from build123d import *

# Parameters (mm, degrees)
BOSS_EXTRUDE1_DEPTH      = 10
BOSS_EXTRUDE1_DEPTH_BACK = 0.01
SKETCH3_W                = 38
SKETCH3_H                = 54
CUT_EXTRUDE1_DEPTH       = 3
SKETCH5_W                = 38
SKETCH5_H                = 54
CUT_EXTRUDE3_DEPTH       = 3
SKETCH15_W               = 20
SKETCH15_H               = 50
BOSS_EXTRUDE3_DEPTH      = 20.3
SKETCH21_R               = 9
CUT_EXTRUDE21_DEPTH      = 20
SKETCH28_W               = 4.75290021
SKETCH28_H               = 9.947843747
BOSS_EXTRUDE6_DEPTH      = 115.870057685
SKETCH30_W               = 14.12
SKETCH30_H               = 25
CUT_EXTRUDE25_DEPTH      = 4.5
SKETCH33_R               = 1.55
CUT_EXTRUDE26_DEPTH      = 10.01
SKETCH36_W               = 38
SKETCH36_H               = 2
BOSS_EXTRUDE7_DEPTH      = 37
SKETCH39_R               = 6
SKETCH39_R_2             = 1.55
CUT_EXTRUDE28_DEPTH      = 2
SKETCH42_R               = 6
SKETCH42_R_2             = 1.55
CUT_EXTRUDE29_DEPTH      = 2
BOSS_EXTRUDE8_REACH      = 265.623
SKETCH44_W               = 25.175895627
SKETCH44_H               = 35.827236085


with BuildPart() as part:
    # Sketch1 → Boss-Extrude1 (new, two sides: drawn at the far end of the back side and taken through both)
    with BuildSketch(Plane.XY.offset(-BOSS_EXTRUDE1_DEPTH_BACK)):
        with BuildLine():
            Line((0, 0), (0, -37))
            Line((0, -37), (60, -37))
            Line((60, -37), (60, -52))
            Line((60, -52), (33.129942315, -78.870057685))
            Line((33.129942315, -78.870057685), (-55.850057685, -78.870057685))
            ThreePointArc((-55.850057685, -78.870057685), (-169.614041234, -90.257166815), (-239.999947532, -0.158696229))
            ThreePointArc((-239.999947532, -0.158696229), (-169.748285548, 90.207490359), (-55.850057685, 78.870057685))
            Line((-55.850057685, 78.870057685), (33.129942315, 78.870057685))
            Line((33.129942315, 78.870057685), (60, 52))
            Line((60, 52), (60, 37))
            Line((60, 37), (0, 37))
            Line((0, 37), (0, 0))
        make_face()
    extrude(amount=BOSS_EXTRUDE1_DEPTH + BOSS_EXTRUDE1_DEPTH_BACK)

    # Sketch3 → Cut-Extrude1 (cut)
    with BuildSketch(Plane.XY.offset(10)):
        with Locations((-19, 51.870057685)):
            Rectangle(SKETCH3_W, SKETCH3_H)
    extrude(amount=-CUT_EXTRUDE1_DEPTH, mode=Mode.SUBTRACT)

    # Sketch5 → Cut-Extrude3 (cut)
    with BuildSketch(Plane.XY.offset(10)):
        with Locations((-19, -51.870057685)):
            Rectangle(SKETCH5_W, SKETCH5_H)
    extrude(amount=-CUT_EXTRUDE3_DEPTH, mode=Mode.SUBTRACT)

    # Sketch15 → Boss-Extrude3 (add)
    with BuildSketch(Plane.XY.offset(10)):
        with Locations((-10, 0.20156489)):
            Rectangle(SKETCH15_W, SKETCH15_H)
    extrude(amount=BOSS_EXTRUDE3_DEPTH)

    # Sketch21 → Cut-Extrude21 (cut)
    with BuildSketch(Plane(origin=(0, 0, 0), x_dir=(0, 0, -1), z_dir=(1, 0, 0))):
        with Locations((-19.36187505, 12.37175029)):
            Circle(SKETCH21_R)
        with Locations((-19.26539558, -14.62824971)):
            Circle(SKETCH21_R)
        with BuildLine():
            Line((-9.491579533, 2.276446619), (-9.557448357, -4.178698144))
            ThreePointArc((-9.557448357, -4.178698144), (-12.081396215, -6.651657156), (-14.554355227, -4.127709299))
            Line((-14.554355227, -4.127709299), (-14.488486403, 2.327435464))
            ThreePointArc((-14.488486403, 2.327435464), (-11.964538545, 4.800394476), (-9.491579533, 2.276446619))
        make_face()
    extrude(amount=-CUT_EXTRUDE21_DEPTH, mode=Mode.SUBTRACT)

    # Sketch28 → Boss-Extrude6 (add)
    with BuildSketch(Plane.XZ.offset(78.870057685)):
        with Locations((16.603067585, 5.033719824)):
            Rectangle(SKETCH28_W, SKETCH28_H)
    extrude(amount=-BOSS_EXTRUDE6_DEPTH)

    # Sketch30 → Cut-Extrude25 (cut)
    with BuildSketch(Plane(origin=(0, 0, -0.01), x_dir=(-1, 0, 0), z_dir=(0, 0, -1))):
        with Locations((-7.06, -49.5)):
            Rectangle(SKETCH30_W, SKETCH30_H)
        Polygon((-14.38072485, 61.935396467), (-14.275539526, 36.935617747), (-0.155664505, 36.995026418), (-0.260849829, 61.994805138), align=None)
    extrude(amount=-CUT_EXTRUDE25_DEPTH, mode=Mode.SUBTRACT)

    # Sketch33 → Cut-Extrude26 (cut)
    with BuildSketch(Plane(origin=(0, 0, -0.01), x_dir=(-1, 0, 0), z_dir=(0, 0, -1))):
        with Locations((-7.06, -53.4)):
            Circle(SKETCH33_R)
        with Locations((-7.06, -49.4)):
            Circle(SKETCH33_R)
        with Locations((-7.06, -45.4)):
            Circle(SKETCH33_R)
        with Locations((-7.06, -41.4)):
            Circle(SKETCH33_R)
        with Locations((-7.228632788, 41.370889137)):
            Circle(SKETCH33_R)
        with Locations((-7.244931474, 45.370855931)):
            Circle(SKETCH33_R)
        with Locations((-7.261230159, 49.370822725)):
            Circle(SKETCH33_R)
        with Locations((-7.277528845, 53.370789519)):
            Circle(SKETCH33_R)
    extrude(amount=-CUT_EXTRUDE26_DEPTH, mode=Mode.SUBTRACT)

    # Sketch36 → Boss-Extrude7 (add)
    with BuildSketch(Plane.XY.offset(7)):
        Polygon((0.279518574, 78.814629504), (0.272425555, 76.814642082), (-37.727335467, 76.949409435), (-37.720242449, 78.949396858), align=None)
        with Locations((-19, -77.815125164)):
            Rectangle(SKETCH36_W, SKETCH36_H)
    extrude(amount=BOSS_EXTRUDE7_DEPTH)

    # Sketch39 → Cut-Extrude28 (cut)
    with BuildSketch(Plane.XZ.offset(78.815125164)):
        with Locations(Location((-19, 19, 0), (0, 0, 270))):
            Circle(SKETCH39_R)
        with Locations(Location((-34.499611559, 25.01055106, 0), (0, 0, 270))):
            Circle(SKETCH39_R_2)
        with Locations(Location((-3.563871147, 24.988758691, 0), (0, 0, 270))):
            Circle(SKETCH39_R_2)
        with Locations(Location((-28.819186805, 37.01055106, 0), (0, 0, 270))):
            Circle(SKETCH39_R_2)
        with Locations(Location((-9.177448314, 36.988758691, 0), (0, 0, 270))):
            Circle(SKETCH39_R_2)
        with Locations(Location((-28.819994175, 13.01055106, 0), (0, 0, 270))):
            Circle(SKETCH39_R_2)
        with Locations(Location((-9.230494356, 12.988758691, 0), (0, 0, 270))):
            Circle(SKETCH39_R_2)
    extrude(amount=-CUT_EXTRUDE28_DEPTH, mode=Mode.SUBTRACT)

    # Sketch42 → Cut-Extrude29 (cut)
    with BuildSketch(Plane(origin=(0.279518574, 78.814629504, 0), x_dir=(0.9999937111161443, -0.003546509292438372, 0), z_dir=(0.003546509292438372, 0.9999937111161443, 0))):
        with Locations(Location((-19.279713392, -19, 0), (0, 0, 180))):
            Circle(SKETCH42_R)
        with Locations(Location((-29.070149337, -13, 0), (0, 0, 180))):
            Circle(SKETCH42_R_2)
        with Locations(Location((-3.778432466, -25, 0), (0, 0, 180))):
            Circle(SKETCH42_R_2)
        with Locations(Location((-9.464104196, -13, 0), (0, 0, 180))):
            Circle(SKETCH42_R_2)
        with Locations(Location((-34.772326096, -25, 0), (0, 0, 180))):
            Circle(SKETCH42_R_2)
        with Locations(Location((-29.096493177, -37, 0), (0, 0, 180))):
            Circle(SKETCH42_R_2)
        with Locations(Location((-9.473371075, -37, 0), (0, 0, 180))):
            Circle(SKETCH42_R_2)
    extrude(amount=-CUT_EXTRUDE29_DEPTH, mode=Mode.SUBTRACT)

    # Boss-Extrude8: up to this face of the body (flat: up to its plane)
    boss_extrude8_end = Plane(part.part.faces().sort_by_distance((26.749098796, 56.040998738, 10))[0])
    # Sketch44 → Boss-Extrude8 (add, up to the picked face)
    with BuildSketch(Plane(origin=(0, 0, -0.01), x_dir=(-1, 0, 0), z_dir=(0, 0, -1)), mode=Mode.PRIVATE) as boss_extrude8_sk1:
        with Locations((-4.733214954, -1.084100606)):
            Rectangle(SKETCH44_W, SKETCH44_H)
    boss_extrude8_tool1 = split(extrude(boss_extrude8_sk1.sketch, amount=-BOSS_EXTRUDE8_REACH, mode=Mode.PRIVATE), bisect_by=boss_extrude8_end, keep=Keep.BOTH, mode=Mode.PRIVATE)
    add(boss_extrude8_tool1.solids().sort_by(Axis((4.733215, -1.084101, -0.01), (0, 0, 1)))[0])


solid = part.part
The model under review builds one solid part; all positions refer to its coordinate system, in mm. A direction names the side the tool comes from. Round coordinates to 2 decimals unless told otherwise and drop trailing zeros. Write each loop counter-clockwise with the first axis right and the second up, starting at its lowest first coordinate (ties: lowest second). Pieces come first, ordered by that corner, then holes. Notation, with made-up numbers: (71, 76) - (102, 76) arc R19 ccw to (102, 95) - close; hole circle Ø3 at (-27.5, 54). An arc over 180 degrees is marked (long way). One line per item, written item: value. Start each with the question number.
1. Consider section C-C on x = -151. Write out the cut boundary in (y, z).
2. To check wall thickness, follow L1, parallel to Y at x = -25, z = 36; L2, parallel to Z at x = -156, y = -70.5; L3, parallel to Y at x = -1.5, z = 16. State the ranges of each line that lie inside material, in increasing order. Write a range as from..to.
3. Consider section B-B on y = 72. Write out the cut boundary in (x, z).
4. The part is to be moulded in two halves that separate along Z. For faces 6 (the face through (9, -49, 4.49)), 7 (the face through (-9.86, -14.233, 28.257)), 8 (the face through (36, -37, 5)), say which applies: released by +Z, released by -Z, zero draft, split by the parting line, or undercut.
5. Consider section A-A on z = 19. Write out the cut boundary in (x, y).
6. Machinability: for faces 1 (the face through (-11, -78.87, 4)), 2 (the face through (37, 37, 5)), 3 (the face through (-19, -50, 7)), 4 (the face through (6, -1, 10)), 5 (the face through (7, 37, 7)), which of the approach directions +Z, -Z, +X, -X, +Y, -Y give a long, thin tool a straight path to every point of the face, cutting with its end or side? Answer none if there is none.
7. Consider section D-D on x = -204. Write out the cut boundary in (y, z), and give its area (3 significant figures).
8. Clearance check with flat-ended pins moving along their axes: P1, Ø9, axis at y = 11, z = 13.5, coming from the +X side; P2, Ø3.5, axis at x = 7.06, y = -49.4, coming from the +Z side; P3, Ø3, axis at x = 36, z = 6, coming from the -Y side; P4, Ø6, axis at y = 7.5, z = 21, coming from the -X side. State where each tip first meets the part, or that it passes through.
Checks:
1. outline: (-96.45, -0.01) - (96.46, -0.01) - (96.46, 10) - (-96.45, 10) - close
2. L1: y = -78.82..-76.82, 76.9..78.9
2. L2: z = -0.01..10
2. L3: y = -78.82..-76.82, -24.8..-23.01, -6.24..4.02, 20.72..25.2, 76.82..78.82
3. outline: (-199.28, -0.01) - (40, -0.01) - (40, 10) - (0, 10) - (0, 7) - (-38, 7) - (-38, 10) - (-199.28, 10) - close
4. face 6: released by -Z
4. face 7: undercut
4. face 8: zero draft
5. outline: (-38, -78.82) - (-25, -78.82) - (-25, -76.82) - (-38, -76.82) - close; (-37.73, 76.95) - (-25.01, 76.9) - (-25, 78.9) - (-37.72, 78.95) - close; (-20, -24.8) - (0, -24.8) - (0, -23.62) - (-20, -23.62) - close; (-20, -5.63) - (0, -5.63) - (0, 3.38) - (-20, 3.38) - close; (-20, 21.36) - (0, 21.36) - (0, 25.2) - (-20, 25.2) - close; (-13.01, 76.86) - (0.27, 76.81) - (0.28, 78.81) - (-13, 78.86) - close; (-13, -78.82) - (0, -78.82) - (0, -76.82) - (-13, -76.82) - close
6. face 1: +Z, -Z, +X, -Y
6. face 2: +Z, -Z, +X
6. face 3: +Z
6. face 4: +X
6. face 5: +Z, -Z
7. outline: (-67.82, -0.01) - (67.81, -0.01) - (67.81, 10) - (-67.82, 10) - close
7. area: 1,360 mm^2
8. P1: stops at x = 18.98
8. P2: stops at z = 10
8. P3: stops at y = -77.5
8. P4: passes through
